Design review of the part built by this model. Coordinates are the model's own, in mm. A direction names the side the tool comes from. Give positions to 0.01 mm unless a question says otherwise; leave off trailing zeros. Write each loop counter-clockwise with the first axis right and the second up, starting at its lowest first coordinate (ties: lowest second). Pieces come first, ordered by that corner, then holes. Notation, with made-up numbers: (18, -7) -> (76, -7) arc R13 cw to (76, -1) -> close; hole circle Ø1 at (-21.75, 47). An arc over 180 degrees is marked (long way). Use CSV: the item, a comma, the result in double quotes.
```python
from build123d import *

# Parameters (mm, degrees)
SKETCH1_R               = 11.1
BOSS_EXTRUDE1_DEPTH     = 4
SKETCH2_R               = 5
BOSS_EXTRUDE2_DEPTH     = 10
BOSS_EXTRUDE3_START     = 1.5
SKETCH3_R               = 5
BOSS_EXTRUDE3_DEPTH     = 1.5
CUT_EXTRUDE1_DEPTH      = 23.06059836
CUT_EXTRUDE1_DEPTH_BACK = 23.06059836
SKETCH4_R               = 4
CUT_EXTRUDE2_DEPTH      = 19.612361484
CUT_EXTRUDE2_DEPTH_BACK = 19.612361484
SKETCH5_R               = 2


with BuildPart() as part:
    # Sketch1 → Boss-Extrude1 (new body)
    with BuildSketch(Plane(origin=(0, 0, 0), x_dir=(0, 0, -1), z_dir=(1, 0, 0))):
        Circle(SKETCH1_R)
    extrude(amount=BOSS_EXTRUDE1_DEPTH)

    # Sketch2 → Boss-Extrude2 (add)
    with BuildSketch(Plane(origin=(4, 0, 0), x_dir=(0, 0, -1), z_dir=(1, 0, 0))):
        Circle(SKETCH2_R)
    extrude(amount=BOSS_EXTRUDE2_DEPTH)

    # Sketch3 → Boss-Extrude3 (add)
    with BuildSketch(Plane.ZY.offset(BOSS_EXTRUDE3_START)):
        with Locations(Location((0, 0, 0), (0, 0, 180))):
            Circle(SKETCH3_R)
    extrude(amount=-BOSS_EXTRUDE3_DEPTH)

    # Sketch4 → Cut-Extrude1 (cut, two sides: drawn at the far end of the back side and taken through both)
    with BuildSketch(Plane.ZY.offset(1.5).offset(-CUT_EXTRUDE1_DEPTH_BACK)):
        Circle(SKETCH4_R)
    extrude(amount=CUT_EXTRUDE1_DEPTH + CUT_EXTRUDE1_DEPTH_BACK, mode=Mode.SUBTRACT)

    # Sketch5 → Cut-Extrude2 (cut, two sides: drawn at the far end of the back side and taken through both)
    with BuildSketch(Plane(origin=(4, 0, 0), x_dir=(0, 0, -1), z_dir=(1, 0, 0)).offset(-CUT_EXTRUDE2_DEPTH_BACK)):
        with Locations((0, 8)):
            Circle(SKETCH5_R)
        with Locations((8, 0)):
            Circle(SKETCH5_R)
        with Locations((0, -8)):
            Circle(SKETCH5_R)
        with Locations((-8, 0)):
            Circle(SKETCH5_R)
    extrude(amount=CUT_EXTRUDE2_DEPTH + CUT_EXTRUDE2_DEPTH_BACK, mode=Mode.SUBTRACT)


solid = part.part
```
(1) Mouldability with a two-part tool opening along Z and no side actions: class faces 1 (the face through (1.97, 9.36, -5.97)), 2 (the face through (4, -2, -5)), 3 (the face through (2, -6, 0)) as +Z half, -Z half, draft (parallel to the pull), parting line (faces both ways), or undercut.
Established:
face 1,"parting line"
face 2,"draft"
face 3,"undercut"
(2) Tool access review of faces 4 (the face through (6.358, -3.905, -0.867)), 5 (the face through (-1, 0, 5)), 6 (the face through (8.93, -4.88, 1.08)): name each direction out of +Z, -Z, +X, -X, +Y, -Y from which nothing blocks a thin tool from reaching the whole face with its end or side.
Established:
face 4,"+X, -X"
face 5,"-X"
face 6,"+X"
(3) Take a section at C-C (y = 8). Write out the cut boundary in (x, z), then the cut area to 3 significant figures.
Established:
outline,"(0, -7.69) -> (4, -7.69) -> (4, -2) -> (0, -2) -> close; (0, 2) -> (4, 2) -> (4, 7.69) -> (0, 7.69) -> close"
area,"45.6 mm2"
(4) Clearance check with flat-ended pins moving along their axes: pin 1 (1.5 mm diameter, centred on x = 6, y = 0, fed in from -Z); pin 2 (5 mm diameter, centred on y = 8, z = 0, fed in from +X); pin 3 (3 mm diameter, centred on x = 11, z = -4.5, fed in from +Y). State where each tip first meets the part, or that it passes through.
Established:
pin 1,"stops at z = -5"
pin 2,"stops at x = 4"
pin 3,"stops at y = 4"
(5) Take a section at A-A (y = 0). Write out the cut boundary in (x, z).
Established:
outline,"(-1.5, -5) -> (0, -5) -> (0, -6) -> (4, -6) -> (4, -5) -> (14, -5) -> (14, -4) -> (-1.5, -4) -> close; (-1.5, 4) -> (14, 4) -> (14, 5) -> (4, 5) -> (4, 6) -> (0, 6) -> (0, 5) -> (-1.5, 5) -> close; (0, -11.1) -> (4, -11.1) -> (4, -10) -> (0, -10) -> close; (0, 10) -> (4, 10) -> (4, 11.1) -> (0, 11.1) -> close"
(6) Take a section at B-B (z = -8.5). Write out the cut boundary in (x, y).
Established:
outline,"(0, -7.14) -> (4, -7.14) -> (4, -1.94) -> (0, -1.94) -> close; (0, 1.94) -> (4, 1.94) -> (4, 7.14) -> (0, 7.14) -> close"
(7) For line 1 along Y through (x, z) = (3.15, 0); line 2 along Y through (x, z) = (2.3, -8); line 3 along X through (y, z) = (8, 4), list the stretches that pass through material, from the lowest coordinate up. Write a range as [from, to].
Established:
line 1,"y = [-11.1, -10], [-6, -4], [4, 6], [10, 11.1]"
line 2,"y = [-7.69, -2], [2, 7.69]"
line 3,"x = [0, 4]"
(8) Take a section at D-D (x = 12). Write out the cut boundary in (y, z), then the cut area to 3 significant figures.
Established:
outline,"circle Ø10 at (0, 0); hole circle Ø8 at (0, 0)"
area,"28.3 mm2"
